from build123d import *

# Parameters (mm, degrees)
SKETCH_1_W          = 50
SKETCH_1_H          = 45
SKETCH_1_R          = 1.65
SKETCH_1_R_2        = 13
EXTRUDE_1_DEPTH     = 6
SKETCH_3_W          = 50
SKETCH_3_H          = 60
EXTRUDE_2_DEPTH     = 6
EXTRUDE_3_DEPTH     = 3
SKETCH_5_R          = 1.6
CUT_EXTRUDE_1_DEPTH = 80.056941504
SKETCH_6_R          = 3.5
CUT_EXTRUDE_2_DEPTH = 2


with BuildPart() as part:
    # 草图1 → 凸台-拉伸1 (new body)
    with BuildSketch(Plane(origin=(0, 0, 0), x_dir=(1, 0, 0), z_dir=(0, 1, 0))):
        with Locations((0, 1.3)):
            Rectangle(SKETCH_1_W, SKETCH_1_H)
        with Locations(Location((-15.5, 15.5, 0), (0, 0, 270))):
            Circle(SKETCH_1_R, mode=Mode.SUBTRACT)
        with Locations(Location((15.5, 15.5, 0), (0, 0, 270))):
            Circle(SKETCH_1_R, mode=Mode.SUBTRACT)
        with Locations(Location((15.5, -15.5, 0), (0, 0, 270))):
            Circle(SKETCH_1_R, mode=Mode.SUBTRACT)
        with Locations(Location((-15.5, -15.5, 0), (0, 0, 270))):
            Circle(SKETCH_1_R, mode=Mode.SUBTRACT)
        with Locations(Location((0, 0, 0), (0, 0, 270))):
            Circle(SKETCH_1_R_2, mode=Mode.SUBTRACT)
    extrude(amount=EXTRUDE_1_DEPTH)

    # 草图3 → 凸台-拉伸2 (add)
    with BuildSketch(Plane.XY.offset(21.2)):
        with Locations((0, 30)):
            Rectangle(SKETCH_3_W, SKETCH_3_H)
    extrude(amount=EXTRUDE_2_DEPTH)

    # 草图4 → 凸台-拉伸3 (add)
    with BuildSketch(Plane.ZY.offset(25)):
        Polygon((-23.8, 6), (21.2, 51), (21.2, 6), align=None)
    extrude_3 = extrude(amount=-EXTRUDE_3_DEPTH)

    # 镜向1: 凸台-拉伸3 across plane
    add(extrude_3.mirror(Plane(origin=(0, 0, 0), x_dir=(0, 0, 1), z_dir=(1, 0, 0))))

    # 草图5 → 切除-拉伸1 (cut, through all)
    with BuildSketch(Plane(origin=(0, 0, 21.2), x_dir=(-1, 0, 0), z_dir=(0, 0, -1))):
        with Locations((-12.5, 46)):
            Circle(SKETCH_5_R)
        with Locations((-12.5, 14)):
            Circle(SKETCH_5_R)
        with Locations(Location((12.5, 14, 0), (0, 0, 180))):
            Circle(SKETCH_5_R)
        with Locations(Location((12.5, 46, 0), (0, 0, 180))):
            Circle(SKETCH_5_R)
    extrude(amount=-CUT_EXTRUDE_1_DEPTH, mode=Mode.SUBTRACT)

    # 草图6 → 切除-拉伸2 (cut)
    with BuildSketch(Plane(origin=(0, 0, 21.2), x_dir=(-1, 0, 0), z_dir=(0, 0, -1))):
        with Locations((-12.5, 46)):
            Circle(SKETCH_6_R)
        with Locations((12.5, 46)):
            Circle(SKETCH_6_R)
        with Locations((-12.5, 14)):
            Circle(SKETCH_6_R)
        with Locations((12.5, 14)):
            Circle(SKETCH_6_R)
    extrude(amount=-CUT_EXTRUDE_2_DEPTH, mode=Mode.SUBTRACT)


solid = part.part
The listing builds one solid part. Answer for the finished solid, in the listing's coordinates (mm). A direction names the side the tool comes from. Give positions to 0.01 mm unless a question says otherwise; leave off trailing zeros. Order: outer loops, then holes, each group sorted by start corner. A loop starts at its lowest first (then second) coordinate and runs counter-clockwise, first axis right, second up. Notation, with made-up numbers: (81, -19) -> (113, -19) arc R19 ccw to (113, -13) -> close; hole circle Ø9 at (72, -30). An arc over 180 degrees is marked (long way). Put each result on its own line as item: value.
Item 1: Given P1, Ø4, axis at x = 15.5, z = -15.5, coming from the +Y side; P2, Ø22.5, axis at y = 37.5, z = -9.5, coming from the +X side; P3, Ø2, axis at x = 11, y = 46, coming from the -Z side; P4, Ø11, axis at x = -12.5, y = 14, coming from the -Z side, each flat-ended and moving along its own axis, determine where each tip first touches the part or whether it passes through.
Established:
P1: stops at y = 6
P2: passes through
P3: stops at z = 23.2
P4: stops at z = 21.2
Item 2: A cutting plane is placed at D-D on y = 5. Give the vertices of the cut face in (x, z).
Established:
outline: (-25, -23.8) -> (25, -23.8) -> (25, 27.2) -> (-25, 27.2) -> close; hole circle Ø3.3 at (-15.5, -15.5); hole circle Ø3.3 at (-15.5, 15.5); hole circle Ø26 at (0, 0); hole circle Ø3.3 at (15.5, -15.5); hole circle Ø3.3 at (15.5, 15.5)
Item 3: For a pull along Y with two mould halves and no side action, classify faces 1 (the face through (-23.5, 28.2, -1.6)), 2 (the face through (-12.04, 49.47, 22.19)), 3 (the face through (-25, 17, 8)) as released by +Y, released by -Y, zero draft, split by the parting line, or undercut.
Established:
face 1: released by +Y
face 2: undercut
face 3: zero draft
Item 4: A cutting plane is placed at C-C on z = 6.5. Give the vertices of the cut face in (x, y), plus the area to 3 significant figures.
Established:
outline: (-25, 0) -> (-11.26, 0) -> (-11.26, 6) -> (-22, 6) -> (-22, 36.3) -> (-25, 36.3) -> close; (11.26, 0) -> (25, 0) -> (25, 36.3) -> (22, 36.3) -> (22, 6) -> (11.26, 6) -> close
area: 347 mm^2
Item 5: A cutting plane is placed at B-B on y = 46. Give the vertices of the cut face in (x, z), plus the area to 3 significant figures.
Established:
outline: (-25, 16.2) -> (-22, 16.2) -> (-22, 21.2) -> (-16, 21.2) -> (-16, 23.2) -> (-14.1, 23.2) -> (-14.1, 27.2) -> (-25, 27.2) -> close; (-10.9, 23.2) -> (-9, 23.2) -> (-9, 21.2) -> (9, 21.2) -> (9, 23.2) -> (10.9, 23.2) -> (10.9, 27.2) -> (-10.9, 27.2) -> close; (14.1, 23.2) -> (16, 23.2) -> (16, 21.2) -> (22, 21.2) -> (22, 16.2) -> (25, 16.2) -> (25, 27.2) -> (14.1, 27.2) -> close
area: 276 mm^2
Item 6: A cutting plane is placed at A-A on x = 5. Give the vertices of the cut face in (y, z).
Established:
outline: (0, -23.8) -> (6, -23.8) -> (6, -12) -> (0, -12) -> close; (0, 12) -> (6, 12) -> (6, 21.2) -> (60, 21.2) -> (60, 27.2) -> (0, 27.2) -> close
Item 7: For faces 4 (the face through (14.868, 2.958, -13.976)), 5 (the face through (-14, 13, 23.2)), 6 (the face through (-22, 19, 9)), determine the directions among +Z, -Z, +X, -X, +Y, -Y from which every point of the face is accessible in a straight line to the end or side of a thin tool.
Established:
face 4: +Y, -Y
face 5: -Z
face 6: -Z, +Y
Item 8: Straight lines are drawn through the part: line 1 (X direction, y = 2.6, z = 15.5); line 2 (Y direction, x = -12.5, z = 22.1); line 3 (Y direction, x = -12.5, z = 25.35). For each, find the intervals that lie inside material, in ascending order.
Established:
line 1: x = -25 to -17.15, -13.85 to 13.85, 17.15 to 25
line 2: y = 0 to 10.5, 17.5 to 42.5, 49.5 to 60
line 3: y = 0 to 12.4, 15.6 to 44.4, 47.6 to 60
